Read the model definition and answer for the solid it produces. Units are mm, in the model's axes. Face numbers are marked on the shaded views. A direction names the side the tool comes from. Give positions to 0.01 mm unless a question says otherwise; leave off trailing zeros. Loops run counter-clockwise (first coordinate to the right, second up) from the corner with the lowest first, then second, coordinate; pieces in that order, holes last. Notation, with made-up numbers: (73, 48) - (124, 48) arc R19 ccw to (124, 79) - close; hole circle Ø4 at (-36.75, -5.5). An arc over 180 degrees is marked (long way). Use a Markdown table: item, result. Add a question column.
Item 1: A cutting plane is placed at D-D (y = 0). Give the number of separate pieces and of enclosed holes in the cut face, plus the area to 3 significant figures.
Item 2: Each of these flat-tipped pins is pushed along its axis until it touches: P1, Ø4, axis at x = -12.7, y = -12.7, coming from the -Z side; P2, Ø10, axis at y = 8, z = 13, coming from the +X side; P3, Ø5.5, axis at x = 13.5, y = 1, coming from the +Z side; P4, Ø5, axis at x = -12.7, y = 0, coming from the +Z side. Where does it stop, or does it pass through?
Item 3: A cutting plane is placed at C-C (y = 7.5). Determine the outline of the cut face in (x, z) (3 decimals), plus the area to 3 significant figures.
Item 4: Consider probe 1 along X at (y, z) = (12.7, -26.4) (1 decimal); probe 2 along X at (y, z) = (-18, 10.5) (3 decimals). Determine where each line is inside the solid, lowest interval first. Write a range as [from, to].
Item 5: Which of the six approach directions +Z, -Z, +X, -X, +Y, -Y give full straight-line access (tool end or side, diameter ignored) to the marked faces 1 and 2?
Item 6: For a pull along Y with two mould halves and no side action, classify the marked faces 3, 4 and 5 as +Y half, -Y half, draft (parallel to the pull), parting line (faces both ways), or undercut.
Item 7: A cutting plane is placed at A-A (z = -4.5). Determine the outline of the cut face in (x, y) (3 decimals).
Item 8: A cutting plane is placed at B-B (x = 17). Determine the outline of the cut face in (y, z) (3 decimals), plus the area to 3 significant figures.
from build123d import *

# Parameters (mm, degrees)
SKETCH1_W           = 44.85
SKETCH1_H           = 44.85
SKETCH1_W_2         = 38.5
SKETCH1_H_2         = 38.5
BOSS_EXTRUDE1_DEPTH = 19.25
SKETCH2_W           = 44.85
SKETCH2_H           = 44.85
BOSS_EXTRUDE2_DEPTH = 3.175
SKETCH3_W           = 44.85
SKETCH3_H           = 44.85
BOSS_EXTRUDE3_DEPTH = 3.175
SKETCH5_R           = 15.875
CUT_EXTRUDE1_DEPTH  = 68.275
SKETCH8_W           = 44.85
SKETCH8_H           = 44.85
SKETCH8_R           = 2.2225
BOSS_EXTRUDE4_DEPTH = 6.35
SKETCH9_R           = 3.4925
CUT_EXTRUDE4_DEPTH  = 6.35
CUT_EXTRUDE5_REACH  = 62.226
SKETCH10_W          = 38.5
SKETCH10_H          = 38.5
CUT_EXTRUDE3_DEPTH  = 43.822445925
SKETCH11_R          = 15.875
CUT_EXTRUDE6_DEPTH  = 43.822445925


with BuildPart() as part:
    # Sketch1 → Boss-Extrude1 (new, symmetric)
    with BuildSketch(Plane(origin=(0, 0, 0), x_dir=(1, 0, 0), z_dir=(0, 1, 0))):
        Rectangle(SKETCH1_W, SKETCH1_H)
        Rectangle(SKETCH1_W_2, SKETCH1_H_2, mode=Mode.SUBTRACT)
    extrude(amount=BOSS_EXTRUDE1_DEPTH, both=True)

    # Sketch2 → Boss-Extrude2 (add)
    with BuildSketch(Plane(origin=(0, 19.25, 0), x_dir=(1, 0, 0), z_dir=(0, 1, 0))):
        Rectangle(SKETCH2_W, SKETCH2_H)
    extrude(amount=BOSS_EXTRUDE2_DEPTH)

    # Sketch3 → Boss-Extrude3 (add)
    with BuildSketch(Plane.XZ.offset(19.25)):
        Rectangle(SKETCH3_W, SKETCH3_H)
    extrude(amount=BOSS_EXTRUDE3_DEPTH)

    # Sketch5 → Cut-Extrude1 (cut, through all)
    with BuildSketch(Plane(origin=(0, -22.425, -22.425), x_dir=(1, 0, 0), z_dir=(0, 1, 0))):
        with Locations(Location((0, -22.425, 0), (0, 0, 90))):
            Circle(SKETCH5_R)
    extrude(amount=CUT_EXTRUDE1_DEPTH, mode=Mode.SUBTRACT)

    # Sketch8 → Boss-Extrude4 (add)
    with BuildSketch(Plane(origin=(0, 0, -22.425), x_dir=(-1, 0, 0), z_dir=(0, 0, -1))):
        Rectangle(SKETCH8_W, SKETCH8_H)
        with Locations((-12.7, 12.7)):
            Circle(SKETCH8_R, mode=Mode.SUBTRACT)
        with Locations((0, 12.7)):
            Circle(SKETCH8_R, mode=Mode.SUBTRACT)
        with Locations((12.7, 12.7)):
            Circle(SKETCH8_R, mode=Mode.SUBTRACT)
        Circle(SKETCH8_R, mode=Mode.SUBTRACT)
        with Locations((12.7, 0)):
            Circle(SKETCH8_R, mode=Mode.SUBTRACT)
        with Locations((0, -12.7)):
            Circle(SKETCH8_R, mode=Mode.SUBTRACT)
        with Locations((12.7, -12.7)):
            Circle(SKETCH8_R, mode=Mode.SUBTRACT)
        with Locations((-12.7, 0)):
            Circle(SKETCH8_R, mode=Mode.SUBTRACT)
        with Locations((-12.7, -12.7)):
            Circle(SKETCH8_R, mode=Mode.SUBTRACT)
    extrude(amount=BOSS_EXTRUDE4_DEPTH)

    # Sketch9 → Cut-Extrude4 (cut)
    with BuildSketch(Plane.XY.offset(-19.25)):
        with Locations((12.7, 12.7)):
            Circle(SKETCH9_R)
        with Locations((0, 12.7)):
            Circle(SKETCH9_R)
        with Locations((-12.7, 12.7)):
            Circle(SKETCH9_R)
        Circle(SKETCH9_R)
        with Locations((-12.7, 0)):
            Circle(SKETCH9_R)
        with Locations((0, -12.7)):
            Circle(SKETCH9_R)
        with Locations((-12.7, -12.7)):
            Circle(SKETCH9_R)
        with Locations((12.7, 0)):
            Circle(SKETCH9_R)
        with Locations((12.7, -12.7)):
            Circle(SKETCH9_R)
    extrude(amount=-CUT_EXTRUDE4_DEPTH, mode=Mode.SUBTRACT)

    # Sketch10 → Cut-Extrude5 (cut, up to next)
    with BuildSketch(Plane.XY.offset(22.425), mode=Mode.PRIVATE) as cut_extrude5_sk1:
        Rectangle(SKETCH10_W, SKETCH10_H)
    cut_extrude5_tool1 = extrude(cut_extrude5_sk1.sketch, amount=-CUT_EXTRUDE5_REACH, mode=Mode.PRIVATE) & part.part
    add(cut_extrude5_tool1.solids().sort_by_distance((0, 0, 22.425))[0], mode=Mode.SUBTRACT)

    # Sketch7 → Cut-Extrude3 (cut, through all)
    with BuildSketch(Plane.ZY):
        with BuildLine():
            Line((0, 15.875), (25, 15.875))
            Line((25, 15.875), (25, -15.875))
            Line((25, -15.875), (0, -15.875))
            ThreePointArc((0, -15.875), (-15.875, 0), (0, 15.875))
        make_face()
    extrude(amount=-CUT_EXTRUDE3_DEPTH, mode=Mode.SUBTRACT)

    # Sketch11 → Cut-Extrude6 (cut, through all)
    with BuildSketch(Plane(origin=(0, 0, 0), x_dir=(0, 0, -1), z_dir=(1, 0, 0))):
        Circle(SKETCH11_R)
    extrude(amount=-CUT_EXTRUDE6_DEPTH, mode=Mode.SUBTRACT)


solid = part.part
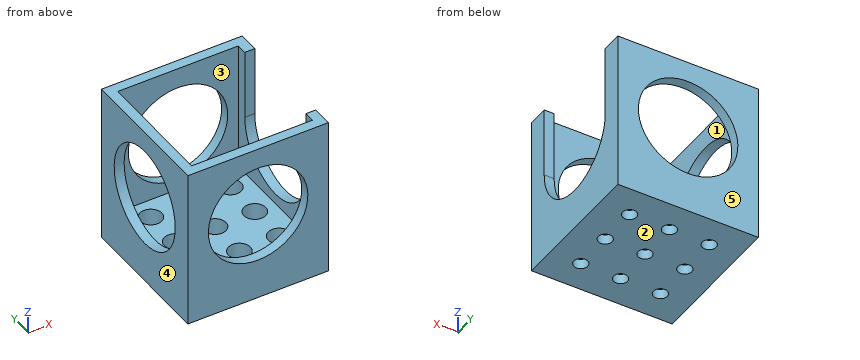
Geometry says:
| question | item | result |
|---|---|---|
| 1 | separate pieces | 5 |
| 1 | enclosed holes | 0 |
| 1 | area | 294 mm² |
| 2 | P1 | through |
| 2 | P2 | x = -19.25 |
| 2 | P3 | z = -19.25 |
| 2 | P4 | z = -25.6 |
| 3 | outline | (-22.425, -28.775) - (22.425, -28.775) - (22.425, -13.992) - (19.25, -13.992) - (19.25, -19.25) - (-19.25, -19.25) - (-19.25, -13.992) - (-22.425, -13.992) - close; (-22.425, 13.992) - (-19.25, 13.992) - (-19.25, 22.425) - (-22.425, 22.425) - close |
| 3 | area | 487 mm² |
| 4 | probe 1 | [-22.4, -14.9], [-10.5, -2.2], [2.2, 10.5], [14.9, 22.4] |
| 4 | probe 2 | [-22.425, -19.25], [19.25, 22.425] |
| 5 | face 1 | +Z |
| 5 | face 2 | -Z, +X, -X, +Y, -Y |
| 6 | face 3 | undercut |
| 6 | face 4 | draft |
| 6 | face 5 | +Y half |
| 7 | outline | (-22.425, -22.425) - (-15.224, -22.425) - (-15.224, -19.25) - (-19.25, -19.25) - (-19.25, -15.224) - (-22.425, -15.224) - close; (-22.425, 15.224) - (-19.25, 15.224) - (-19.25, 19.25) - (-15.224, 19.25) - (-15.224, 22.425) - (-22.425, 22.425) - close; (15.224, -22.425) - (22.425, -22.425) - (22.425, -15.224) - (19.25, -15.224) - (19.25, -19.25) - (15.224, -19.25) - close; (15.224, 19.25) - (19.25, 19.25) - (19.25, 15.224) - (22.425, 15.224) - (22.425, 22.425) - (15.224, 22.425) - close |
| 8 | outline | (-22.425, -28.775) - (22.425, -28.775) - (22.425, 22.425) - (19.25, 22.425) - (19.25, -19.25) - (-19.25, -19.25) - (-19.25, 22.425) - (-22.425, 22.425) - close |
| 8 | area | 692 mm² |
